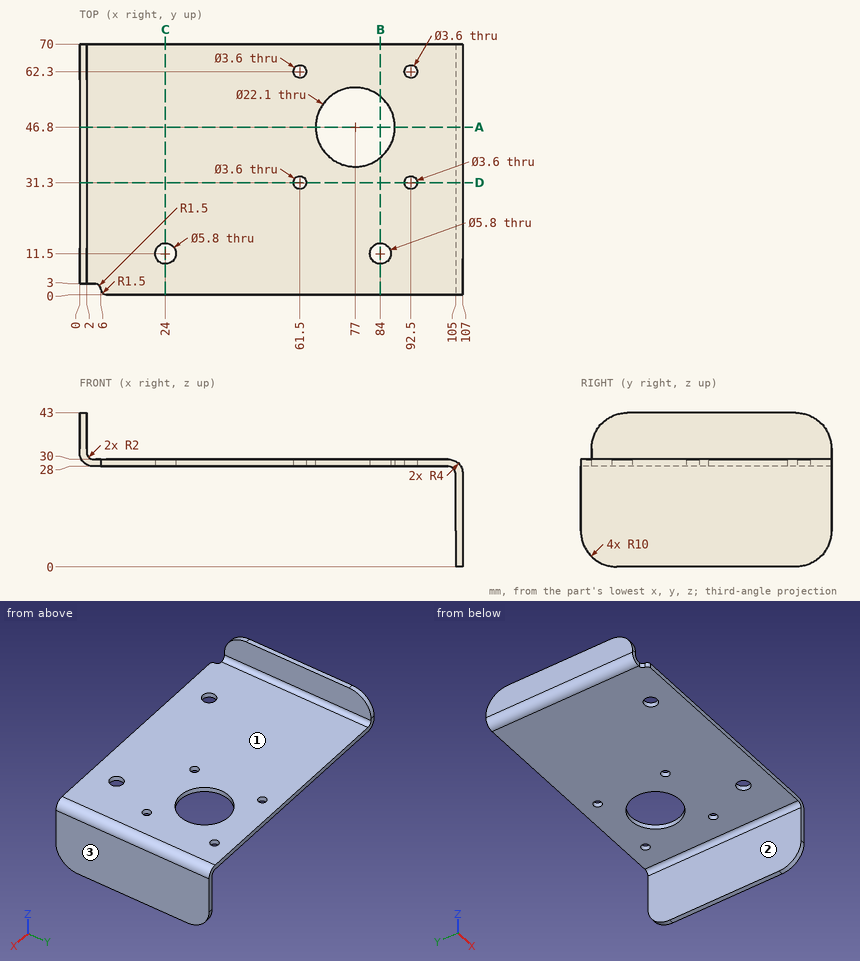
Source: three-view drawing plus pictorial views. Frame: mm from the lowest corner of the part. A direction names the side the tool comes from. Give positions to 0.01 mm unless a question says otherwise; leave off trailing zeros. Order: outer loops, then holes, each group sorted by start corner. A loop starts at its lowest first (then second) coordinate and runs counter-clockwise, first axis right, second up. Notation, with made-up numbers: (-34.75, 23) -> (-20.75, 23) arc R21 ccw to (-20.75, 30) -> close; hole circle Ø1 at (80.25, 53). An arc over 180 degrees is marked (long way). Use a Markdown table: item, result.
Q1. Material intervals for line 1 (Y direction, x = 61.5, z = 29.2); line 2 (Y direction, x = 84, z = 28.9); line 3 (Z direction, x = 82, y = 36), sorted ascending. Write a range as [from, to].
A:
| item | result |
|---|---|
| line 1 | [0, 29.5], [33.1, 60.5], [64.1, 70] |
| line 2 | [0, 8.6], [14.4, 38.25], [55.35, 70] |
| line 3 | [28, 30] |
Q2. Section B-B (x = 84). Return the cut outline in (y, z).
A:
| item | result |
|---|---|
| outline | (0, 28) -> (8.6, 28) -> (8.6, 30) -> (0, 30) -> close; (14.4, 28) -> (38.25, 28) -> (38.25, 30) -> (14.4, 30) -> close; (55.35, 28) -> (70, 28) -> (70, 30) -> (55.35, 30) -> close |
Q3. Section D-D (y = 31.3). Return the cut outline in (x, z).
A:
| item | result |
|---|---|
| outline | (0, 32) arc R4 ccw to (4, 28) -> (59.7, 28) -> (59.7, 30) -> (4, 30) arc R2 cw to (2, 32) -> (2, 43) -> (0, 43) -> close; (63.3, 28) -> (90.7, 28) -> (90.7, 30) -> (63.3, 30) -> close; (94.3, 28) -> (103, 28) arc R2 cw to (105, 26) -> (105, 0) -> (107, 0) -> (107, 26) arc R4 ccw to (103, 30) -> (94.3, 30) -> close |
Q4. Section A-A (y = 46.8). Return the cut outline in (x, z).
A:
| item | result |
|---|---|
| outline | (0, 32) arc R4 ccw to (4, 28) -> (65.95, 28) -> (65.95, 30) -> (4, 30) arc R2 cw to (2, 32) -> (2, 43) -> (0, 43) -> close; (88.05, 28) -> (103, 28) arc R2 cw to (105, 26) -> (105, 0) -> (107, 0) -> (107, 26) arc R4 ccw to (103, 30) -> (88.05, 30) -> close |
Q5. Section C-C (x = 24). Return the cut outline in (y, z), and give its area (3 significant figures).
A:
| item | result |
|---|---|
| outline | (0, 28) -> (8.6, 28) -> (8.6, 30) -> (0, 30) -> close; (14.4, 28) -> (70, 28) -> (70, 30) -> (14.4, 30) -> close |
| area | 128 mm^2 |
Q6. Access query for the marked faces 1, 2 and 3. Directions: +Z, -Z, +X, -X, +Y, -Y. A direction counts if a zero-diameter tool reaches every point of the face in a straight line with its end or side. Return the directions, or none.
A:
| item | result |
|---|---|
| face 1 | +Z, +X, +Y, -Y |
| face 2 | -Z, -X, +Y, -Y |
| face 3 | +Z, -Z, +X, +Y, -Y |
Q7. First-contact query: P1, Ø17.5, axis at x = 77, y = 46.8, coming from the -Z side; P2, Ø4, axis at y = 43, z = 24, coming from the -X side; P3, Ø10, axis at x = 94, y = 57, coming from the -Z side; P4, Ø5, axis at x = 3, z = 29.5, coming from the -Y side. Flat tips, straight axial feed; report the tip coordinate or a pass-through.
A:
| item | result |
|---|---|
| P1 | through |
| P2 | x = 105 |
| P3 | z = 28 |
| P4 | y = 2.62 |
